Verification items for the finished model (mm, model axes). Face numbers are marked on the shaded views. A direction names the side the tool comes from. Coordinates: 2 decimals unless noted, no trailing zeros. Order: outer loops, then holes, each group sorted by start corner. A loop starts at its lowest first (then second) coordinate and runs counter-clockwise, first axis right, second up. Notation, with made-up numbers: M -20.75,84 L -16.75,84 A14 cw -16.75,107 Z; hole C 4,-23 d7. An arc over 180 degrees is marked long. Return JSON: item names as keys, results as strings. Group by question number.
Q1. Mould release check, pull along X, two halves, no side actions. Record for the marked faces 1, 2 and 3: pulls with the +X half, pulls with the -X half, needs draft (parallel to the pull), parting line crosses it, or undercut.
Q2. Access from +Z, -Z, +X, -X, +Y, -Y to the whole of each face (thin tool, end or side, straight path). Record for the marked faces 4 and 5.
Q3. Section check A-A, the plane x = 0. Enter the section's corners in (y, z).
Q4. Section check D-D, the plane x = 10.5. Enter the section's corners in (y, z).
Q5. Go/stop test with flat-tipped pins: pin 1 Ø0.8 at (y, z) = (-1, 2) entering from +X (3 decimals); pin 2 Ø4.5 at (x, y) = (13.5, 0) entering from +Z; pin 3 Ø1.5 at (y, z) = (0.5, 1.5) entering from -X (3 decimals); pin 4 Ø1 at (x, y) = (5, 2.5) entering from -Z. Record where each tip stops, or that it passes through.
Q6. Section check B-B, the plane y = 0. Enter the section's corners in (x, z) (3 decimals), then the cut area to 3 significant figures.
Q7. Thickness scan on probe 1 along Y at (x, z) = (-9, 1.4); probe 2 along X at (y, z) = (1.25, 3) (3 decimals); probe 3 along Y at (x, z) = (11, 1.8). Record the ranges inside material, lowest first.
Q8. Section check C-C, the plane x = 4.5. Enter the section's corners in (y, z).
from build123d import *

# Parameters (mm, degrees)
F0_W         = 3.3528
F0_H         = 2.5146
F0_R         = 0.80645
F1_DEPTH     = 3.048
F2_W         = 2.54
F2_H         = 10.7442
F2_W_2       = 18.796
F2_H_2       = 7.9502
F3_DEPTH     = 1.27
F4_W         = 6.35
F4_H         = 5.715
F5_DEPTH     = 2.54
F6_R         = 0.79375
F7_DEPTH     = 10.7452
F8_DEPTH     = 0.508
F9_W         = 3.81
F9_H         = 2.5146
F10_DEPTH    = 0.762
F11_T1_DEPTH = 10.445747458
F11_T3_DEPTH = 10.445747458
F11_T5_DEPTH = 12.6746
F11_T7_DEPTH = 12.6746
F12_R        = 0.381
F8_FACE_W    = 7.9502
F8_FACE_H    = 1.778
F13_DEPTH    = 1.397


# Not quite as in the source:
# - a fillet or chamfer that OpenCascade refuses, or shapes differently, is made with other operations: its cross-section is extruded or revolved along the edge and cut away or added


with BuildPart() as f1:
    # F0 (on Top) → F1 (new body)
    with BuildSketch(Plane.XY):
        with Locations((-12.4714, 4.1148)):
            Rectangle(F0_W, F0_H)
        with Locations((-12.4714, -4.1148)):
            Rectangle(F0_W, F0_H)
        Polygon((10.795, 5.3721), (-10.795, 5.3721), (-10.795, 2.8575), (-10.795, -2.8575), (-10.795, -5.3721), (10.795, -5.3721), (17.145, -5.3721), (17.145, 5.3721), align=None)
        with Locations((-6.985, 0)):
            Circle(F0_R, mode=Mode.SUBTRACT)
        with BuildLine():
            ThreePointArc((-1.7885716042, 1.644670926), (-2.2375844102, 2.728683732), (-1.1535716042, 2.279670926))
            Line((-1.1535716042, 2.279670926), (1.1535716042, 2.279670926))
            ThreePointArc((1.1535716042, 2.279670926), (2.2375844102, 2.728683732), (1.7885716042, 1.644670926))
            Line((1.7885716042, 1.644670926), (1.7885716042, 0.635))
            ThreePointArc((1.7885716042, 0.635), (2.4235716042, 0), (1.7885716042, -0.635))
            Line((1.7885716042, -0.635), (1.7885716042, -1.644670926))
            ThreePointArc((1.7885716042, -1.644670926), (2.2375844102, -2.728683732), (1.1535716042, -2.279670926))
            Line((1.1535716042, -2.279670926), (-1.1535716042, -2.279670926))
            ThreePointArc((-1.1535716042, -2.279670926), (-2.2375844102, -2.728683732), (-1.7885716042, -1.644670926))
            Line((-1.7885716042, -1.644670926), (-1.7885716042, -0.635))
            ThreePointArc((-1.7885716042, -0.635), (-2.4235716042, 0), (-1.7885716042, 0.635))
            Line((-1.7885716042, 0.635), (-1.7885716042, 1.644670926))
        make_face(mode=Mode.SUBTRACT)
        with Locations((6.985, 0)):
            Circle(F0_R, mode=Mode.SUBTRACT)
    extrude(amount=F1_DEPTH)

    # F2 (on face) → F3 (cut)
    with BuildSketch(Plane.XY.offset(3.048)):
        with Locations((15.875, 0)):
            Rectangle(F2_W, F2_H)
        Rectangle(F2_W_2, F2_H_2)
    extrude(amount=-F3_DEPTH, mode=Mode.SUBTRACT)

    # F4 (on face) → F5 (cut)
    with BuildSketch(Plane.XY.offset(3.048)):
        with Locations((13.97, 0)):
            Rectangle(F4_W, F4_H)
    extrude(amount=-F5_DEPTH, mode=Mode.SUBTRACT)

    # F6 (on face) → F7 (cut, through all)
    with BuildSketch(Plane.XZ.offset(5.3721)):
        with Locations((-12.446, 1.524)):
            Circle(F6_R)
        with Locations((12.5476, 2.159)):
            Circle(F6_R)
    extrude(amount=-F7_DEPTH, mode=Mode.SUBTRACT)

    # F8 (cut): a face of the model
    f8_faces = [f1.faces().sort_by_distance(p)[0] for p in [
        (0, 3.7710178361, 1.778),
    ]]
    extrude(f8_faces, amount=-F8_DEPTH, mode=Mode.SUBTRACT)

    # F9 (on face) → F10 (join)
    with BuildSketch(Plane.XY.offset(3.048)):
        with Locations((12.7, 4.1148)):
            Rectangle(F9_W, F9_H)
        with Locations((12.7, -4.1148)):
            Rectangle(F9_W, F9_H)
    extrude(amount=F10_DEPTH)

    # F11: fillet of radius 2.032 on 4 edges, made by hand

    # F11_s2 → F11_t1 (cut)
    with BuildSketch(Plane.XZ.offset(-1.108073729)):
        with BuildLine():
            ThreePointArc((12.3812294916, 3.81), (11.5013476813, 3.6096200479), (10.795, 3.048))
            Line((10.795, 3.048), (10.795, 3.81))
            Line((10.795, 3.81), (12.3812294916, 3.81))
        make_face()
    extrude(amount=F11_T1_DEPTH, mode=Mode.SUBTRACT)

    # F11_s4 → F11_t3 (cut)
    with BuildSketch(Plane.XZ.offset(-9.337673729)):
        with BuildLine():
            ThreePointArc((12.3812294916, 3.81), (11.5013476813, 3.6096200479), (10.795, 3.048))
            Line((10.795, 3.048), (10.795, 3.81))
            Line((10.795, 3.81), (12.3812294916, 3.81))
        make_face()
    extrude(amount=F11_T3_DEPTH, mode=Mode.SUBTRACT)

    # F11_s6 → F11_t5 (cut)
    with BuildSketch(Plane.XZ.offset(-10.4521)):
        with BuildLine():
            ThreePointArc((14.605, 1.778), (14.0098409794, 3.2148409794), (12.573, 3.81))
            Line((12.573, 3.81), (14.605, 3.81))
            Line((14.605, 3.81), (14.605, 1.778))
        make_face()
    extrude(amount=F11_T5_DEPTH, mode=Mode.SUBTRACT)

    # F11_s8 → F11_t7 (cut)
    with BuildSketch(Plane.XZ.offset(-2.2225)):
        with BuildLine():
            ThreePointArc((14.605, 1.778), (14.0098409794, 3.2148409794), (12.573, 3.81))
            Line((12.573, 3.81), (14.605, 3.81))
            Line((14.605, 3.81), (14.605, 1.778))
        make_face()
    extrude(amount=F11_T7_DEPTH, mode=Mode.SUBTRACT)

    # F12 (on face) + F8_face (on face) → F13 (cut, through all)
    with BuildSketch(Plane(origin=(-10.795, 0, 0), x_dir=(0, -1, 0), z_dir=(-1, 0, 0))):
        with Locations((-0.9525, 2.0008196589)):
            Circle(F12_R)
    with BuildSketch(Plane(origin=(-9.398, 0, 2.159), x_dir=(0, 1, 0), z_dir=(1, 0, 0))):
        Rectangle(F8_FACE_W, F8_FACE_H)
    extrude(amount=-F13_DEPTH, dir=(-1, 0, 0), mode=Mode.SUBTRACT)


solid = f1.part
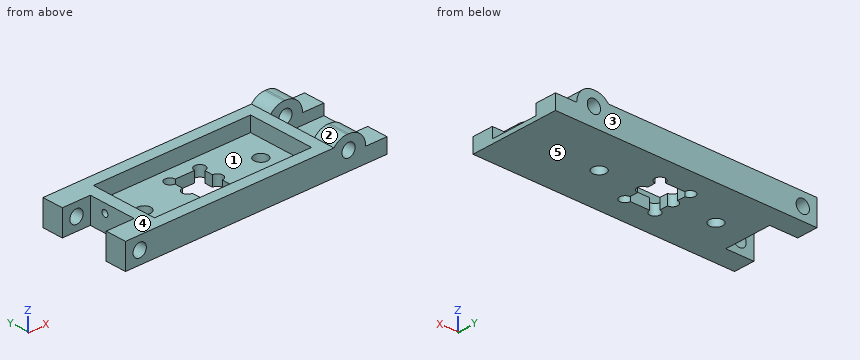
Numbers:
{
 "1": {"face 1": "undercut", "face 2": "pulls with the -X half", "face 3": "needs draft"},
 "2": {"face 4": "+Z, -X, +Y, -Y", "face 5": "-Z, +X, -X, +Y, -Y"},
 "3": {"outline": "M -5.37,0 L -2.28,0 L -2.28,1.27 L -3.98,1.27 L -3.98,3.05 L -5.37,3.05 Z; M 2.28,0 L 5.37,0 L 5.37,3.05 L 3.98,3.05 L 3.98,1.27 L 2.28,1.27 Z"},
 "4": {"outline": "M -5.37,0 L 5.37,0 L 5.37,3.05 L -5.37,3.05 Z"},
 "5": {"pin 1": "stops at x = 10.795", "pin 2": "stops at z = 0.51", "pin 3": "stops at x = -10.795", "pin 4": "stops at z = 0"},
 "6": {"outline": "M -10.795,0 L -7.791,0 L -7.791,1.27 L -9.398,1.27 L -9.398,3.048 L -10.795,3.048 Z; M -6.179,0 L -2.424,0 L -2.424,1.27 L -6.179,1.27 Z; M 2.424,0 L 6.179,0 L 6.179,1.27 L 2.424,1.27 Z; M 7.791,0 L 17.145,0 L 17.145,0.508 L 10.795,0.508 L 10.795,3.048 L 9.398,3.048 L 9.398,1.27 L 7.791,1.27 Z", "area": "25.4 mm2"},
 "7": {"probe 1": "y = -5.37 to -3.98, 3.98 to 5.37", "probe 2": "x = -10.795 to -9.398, 9.398 to 10.795", "probe 3": "y = -5.37 to -2.86, 2.86 to 5.37"},
 "8": {"outline": "M -5.37,0 L 5.37,0 L 5.37,3.05 L 3.98,3.05 L 3.98,1.27 L -3.98,1.27 L -3.98,3.05 L -5.37,3.05 Z"}
}
